```python
from build123d import *

# Parameters (mm, degrees)
SKETCH3_RX          = 27
SKETCH3_RY          = 15
BOSS_EXTRUDE1_DEPTH = 60.053544519
CUT_EXTRUDE1_DEPTH  = 99
BOSS_EXTRUDE2_DEPTH = 3


with BuildPart() as part:
    # Sketch3 → Boss-Extrude1 (new body)
    with BuildSketch(Plane(origin=(0, 0, 0), x_dir=(1, 0, 0), z_dir=(0, 1, 0))):
        with Locations((0, 0)):
            Ellipse(SKETCH3_RX, SKETCH3_RY)
        with BuildLine():
            Line((22.5, 6.5), (22.5, -6.5))
            ThreePointArc((22.5, -6.5), (0, -10.878511347), (-22.5, -6.5))
            Line((-22.5, -6.5), (-22.5, 6.5))
            ThreePointArc((-22.5, 6.5), (0, 10.878511347), (22.5, 6.5))
        make_face(mode=Mode.SUBTRACT)
    extrude(amount=BOSS_EXTRUDE1_DEPTH)

    # Loft9: read off the stored shape, not the designer's step
    # Loft9: loft between two sections, ruled curve by curve
    loft9_from = [
        Edge.make_bspline([(0.559362113, 0, -14.996780663), (-53.429048274, 0, -15.618294122), (-54.5477725, 0, 14.375267204), (-0.559362113, 0, 14.996780663), (53.429048274, 0, 15.618294122), (54.5477725, 0, -14.375267204), (0.559362113, 0, -14.996780663)], [0, 0, 0, 0, 0.5, 0.5, 0.5, 1, 1, 1, 1], 3, [1, 0.333333333, 0.333333333, 1, 0.333333333, 0.333333333, 1]),
    ]
    loft9_to = [
        Edge.make_bspline([(0.162188065, 60.053544519, -31.999588982), (-63.836989899, 60.053544519, -32.323965112), (-64.16136603, 60.053544519, 31.675212852), (-0.162188065, 60.053544519, 31.999588982), (63.836989899, 60.053544519, 32.323965112), (64.16136603, 60.053544519, -31.675212852), (0.162188065, 60.053544519, -31.999588982)], [0, 0, 0, 0, 0.5, 0.5, 0.5, 1, 1, 1, 1], 3, [1, 0.333333333, 0.333333333, 1, 0.333333333, 0.333333333, 1]),
    ]
    loft9 = Solid(Shell([*[Face.make_surface_from_curves(loft9_from[k], loft9_to[k]) for k in range(1)], Face(Wire(loft9_from)), Face(Wire(loft9_to))]))
    add(loft9)

    # Sketch5 → Cut-Extrude1 (cut)
    with BuildSketch(Plane(origin=(0, 60.053544519, 0), x_dir=(1, 0, 0), z_dir=(0, 1, 0))):
        with BuildLine():
            Line((22.5, 6.5), (22.5, -6.5))
            ThreePointArc((22.5, -6.5), (0, -10.878511347), (-22.5, -6.5))
            Line((-22.5, -6.5), (-22.5, 6.5))
            ThreePointArc((-22.5, 6.5), (0, 10.878511347), (22.5, 6.5))
        make_face()
    extrude(amount=-CUT_EXTRUDE1_DEPTH, mode=Mode.SUBTRACT)

    # Sketch5<4> → Boss-Extrude2 (add)
    with BuildSketch(Plane(origin=(0, 60.053544519, 0), x_dir=(1, 0, 0), z_dir=(0, 1, 0))):
        with BuildLine():
            Line((-19.5, -7.621352305), (-19.5, 7.621352305))
            ThreePointArc((-19.5, 7.621352305), (-21.007483375, 7.080696734), (-22.5, 6.5))
            Line((-22.5, 6.5), (-22.5, -6.5))
            ThreePointArc((-22.5, -6.5), (-21.007483375, -7.080696734), (-19.5, -7.621352305))
        make_face()
        with BuildLine():
            Line((22.5, -6.5), (22.5, 6.5))
            ThreePointArc((22.5, 6.5), (21.007483375, 7.080696734), (19.5, 7.621352305))
            Line((19.5, 7.621352305), (19.5, -7.621352305))
            ThreePointArc((19.5, -7.621352305), (21.007483375, -7.080696734), (22.5, -6.5))
        make_face()
    extrude(amount=-BOSS_EXTRUDE2_DEPTH)


solid = part.part
```
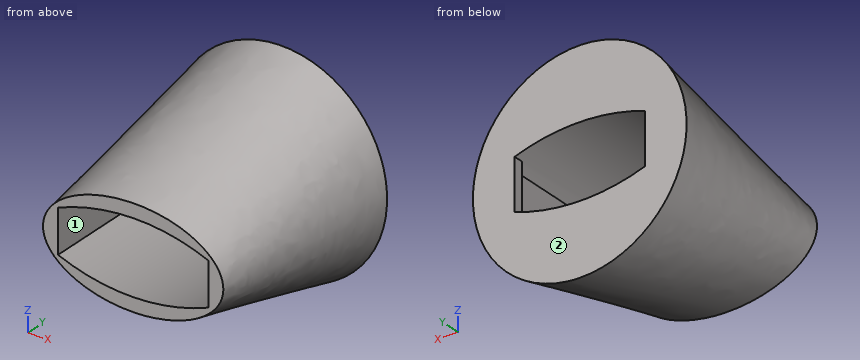
Geometry check sheet. Reference: the model listing, model coordinates, mm. Face numbers are marked on the shaded views. Coordinates: 2 decimals unless noted, no trailing zeros.
Q1. Thickness scan on probe 1 along Z at (x, y) = (5, 37.5); probe 2 along Z at (x, y) = (-3, 38.5); probe 3 along X at (y, z) = (16, 2). Record the ranges inside material, lowest first.
Reply:
probe 1: z = -25.27 to -10.67, 10.67 to 25.25
probe 2: z = -25.77 to -10.8, 10.8 to 25.77
probe 3: x = -28.19 to -22.5, 22.5 to 28.18
Q2. Draft check along Z on the marked faces 1 and 2. Enter one of: released by +Z, released by -Z, zero draft, split by the parting line, or undercut.
Reply:
face 1: undercut
face 2: zero draft
Q3. Depth check by flat-ended pin: pin 1 Ø0.9 at (y, z) = (58, -1) entering from -X; pin 2 Ø3.5 at (y, z) = (58, 0) entering from +X; pin 3 Ø14.5 at (y, z) = (14.5, -1) entering from +X. Enter the tip coordinate at first touch or a pass-through.
Reply:
pin 1: stops at x = -31.85
pin 2: stops at x = 31.97
pin 3: stops at x = 28.81
